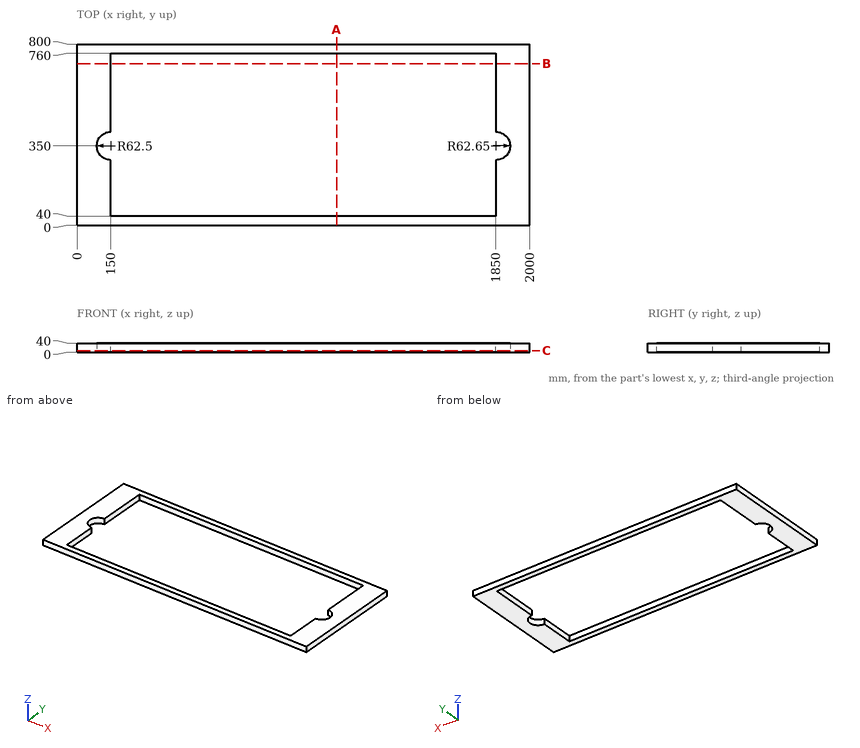
For this review, use the dimensioned drawing (mm, ordinates from the lowest corner) and the shaded views. Round coordinates to 2 decimals unless told otherwise and drop trailing zeros. Order: outer loops, then holes, each group sorted by start corner. A loop starts at its lowest first (then second) coordinate and runs counter-clockwise, first axis right, second up. Notation, with made-up numbers: (-30.75, 25.5) -> (-12.75, 25.5) arc R19 ccw to (-12.75, 35.5) -> close; hole circle Ø8 at (-12, 64.25). An arc over 180 degrees is marked (long way). One line per item, written item: value. Start each with the question number.
Q1. Wall thickness on line 1 (X direction, y = 228, z = 28); line 2 (Y direction, x = 922, z = 37.5); line 3 (X direction, y = 298.5, z = 6): over which ranges is each line inside the solid? List them lowest first.
Q2. Take a section at A-A (x = 1146.5). Write out the cut boundary in (y, z), and give its area (3 significant figures).
Q3. Take a section at B-B (y = 713). Write out the cut boundary in (x, z).
Q4. Take a section at C-C (z = 7). Write out the cut boundary in (x, y).
Reported:
1. line 1: x = 0 to 150, 1850 to 2000
1. line 2: y = 0 to 40, 760 to 800
1. line 3: x = 0 to 114.59, 1885.68 to 2000
2. outline: (0, 0) -> (40, 0) -> (40, 40) -> (0, 40) -> close; (760, 0) -> (800, 0) -> (800, 40) -> (760, 40) -> close
2. area: 3,200 mm2
3. outline: (0, 0) -> (150, 0) -> (150, 40) -> (0, 40) -> close; (1850, 0) -> (2000, 0) -> (2000, 40) -> (1850, 40) -> close
4. outline: (0, 0) -> (2000, 0) -> (2000, 800) -> (0, 800) -> close; hole (150, 40) -> (1850, 40) -> (1850, 287.35) arc R62.65 ccw to (1850, 412.65) -> (1850, 760) -> (150, 760) -> (150, 412.5) arc R62.5 ccw to (150, 287.5) -> close
